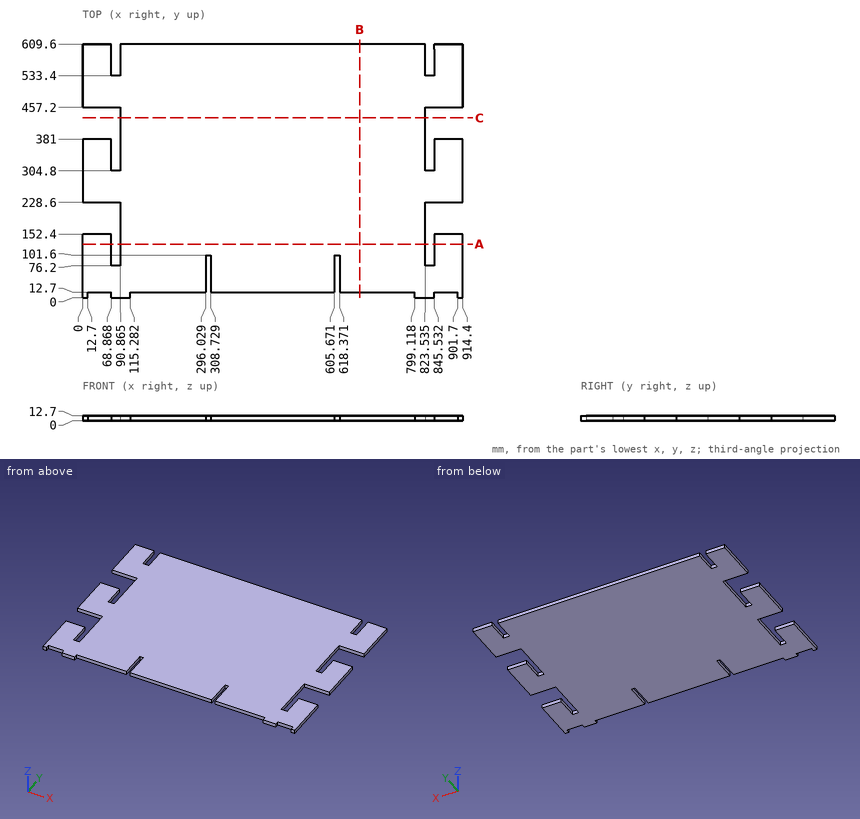
Geometry: see drawing. Coordinates: mm, zero at the bounding-box minimum. Round coordinates to 2 decimals unless told otherwise and drop trailing zeros. Order: outer loops, then holes, each group sorted by start corner. A loop starts at its lowest first (then second) coordinate and runs counter-clockwise, first axis right, second up. Notation, with made-up numbers: (44, -21) - (65, -21) arc R34 cw to (65, 18) - close; hole circle Ø6 at (3.5, -17.5). An arc over 180 degrees is marked (long way). Use a Markdown table: item, result. Add a question column.
1. Section query C-C (y = 432). Return the cut outline in (x, z) (1 decimal).
2. First-contact query: pin 1 (6 mm diameter, centred on x = 794, z = 6.5, fed in from -Y); pin 2 (6.5 mm diameter, centred on x = 78.5, z = 5, fed in from +Y); pin 3 (4 mm diameter, centred on y = 415, z = 4.5, fed in from -X) (1 decimal). Flat tips, straight axial feed; report the tip coordinate or a pass-through.
3. Section query B-B (x = 666). Return the cut outline in (y, z).
4. Section query A-A (y = 128.5). Return the cut outline in (x, z) (1 decimal).
5. Line query: probe 1 along X at (y, z) = (51, 7.5); probe 2 along X at (y, z) = (307, 3.5) (1 decimal); probe 3 along Y at (x, z) = (858.5, 1.5). Output: solid intervals per line, ascending.
Derived:
| question | item | result |
|---|---|---|
| 1 | outline | (90.9, 0) - (823.5, 0) - (823.5, 12.7) - (90.9, 12.7) - close |
| 2 | pin 1 | y = 12.7 |
| 2 | pin 2 | y = 533.4 |
| 2 | pin 3 | x = 90.9 |
| 3 | outline | (12.7, 0) - (609.6, 0) - (609.6, 12.7) - (12.7, 12.7) - close |
| 4 | outline | (0, 0) - (68.9, 0) - (68.9, 12.7) - (0, 12.7) - close; (90.9, 0) - (823.5, 0) - (823.5, 12.7) - (90.9, 12.7) - close; (845.5, 0) - (914.4, 0) - (914.4, 12.7) - (845.5, 12.7) - close |
| 5 | probe 1 | 0 to 296.03, 308.73 to 605.67, 618.37 to 914.4 |
| 5 | probe 2 | 0 to 68.9, 90.9 to 823.5, 845.5 to 914.4 |
| 5 | probe 3 | 12.7 to 152.4, 228.6 to 381, 457.2 to 609.6 |
